```python
from build123d import *

# Parameters (mm, degrees)
SKETCH1_W               = 170
SKETCH1_H               = 80
SKETCH1_W_2             = 140
SKETCH1_H_2             = 50
BOSS_EXTRUDE1_DEPTH     = 20
CUT_EXTRUDE1_DEPTH      = 119.427192823
CUT_EXTRUDE1_DEPTH_BACK = 119.427192823
SKETCH2_R               = 6.3
CUT_EXTRUDE3_REACH      = 98.047
SKETCH5_R               = 2.75
FILLET1_R               = 2
FILLET2_R               = 5
SKETCH6_R               = 6
CUT_EXTRUDE4_DEPTH      = 119.427192823
SKETCH7_R               = 2.75
CUT_EXTRUDE5_DEPTH      = 97.046863561


with BuildPart() as part:
    # Sketch1 → Boss-Extrude1 (new body)
    with BuildSketch(Plane.XY):
        Rectangle(SKETCH1_W, SKETCH1_H)
        Rectangle(SKETCH1_W_2, SKETCH1_H_2, mode=Mode.SUBTRACT)
    extrude(amount=BOSS_EXTRUDE1_DEPTH)

    # Sketch2 → Cut-Extrude1 (cut, two sides: drawn at the far end of the back side and taken through both)
    with BuildSketch(Plane(origin=(0, 40, 0), x_dir=(1, 0, 0), z_dir=(0, 1, 0)).offset(-CUT_EXTRUDE1_DEPTH_BACK)):
        with Locations(Location((-60, -10, 0), (0, 0, 270))):
            Circle(SKETCH2_R)
        with Locations(Location((-10, -10, 0), (0, 0, 270))):
            Circle(SKETCH2_R)
    extrude(amount=CUT_EXTRUDE1_DEPTH + CUT_EXTRUDE1_DEPTH_BACK, mode=Mode.SUBTRACT)

    # Sketch5 → Cut-Extrude3 (cut, up to next)
    with BuildSketch(Plane(origin=(0, 0, 0), x_dir=(-1, 0, 0), z_dir=(0, 0, -1)), mode=Mode.PRIVATE) as cut_extrude3_sk1:
        with Locations((35, 32.5)):
            Circle(SKETCH5_R)
    cut_extrude3_tool1 = extrude(cut_extrude3_sk1.sketch, amount=-CUT_EXTRUDE3_REACH, mode=Mode.PRIVATE) & part.part
    # Sketch5 → Cut-Extrude3 (cut, up to next)
    with BuildSketch(Plane(origin=(0, 0, 0), x_dir=(-1, 0, 0), z_dir=(0, 0, -1)), mode=Mode.PRIVATE) as cut_extrude3_sk2:
        with Locations((35, -32.5)):
            Circle(SKETCH5_R)
    cut_extrude3_tool2 = extrude(cut_extrude3_sk2.sketch, amount=-CUT_EXTRUDE3_REACH, mode=Mode.PRIVATE) & part.part
    # Sketch5 → Cut-Extrude3 (cut, up to next)
    with BuildSketch(Plane(origin=(0, 0, 0), x_dir=(-1, 0, 0), z_dir=(0, 0, -1)), mode=Mode.PRIVATE) as cut_extrude3_sk3:
        with Locations((-5, 32.5)):
            Circle(SKETCH5_R)
    cut_extrude3_tool3 = extrude(cut_extrude3_sk3.sketch, amount=-CUT_EXTRUDE3_REACH, mode=Mode.PRIVATE) & part.part
    # Sketch5 → Cut-Extrude3 (cut, up to next)
    with BuildSketch(Plane(origin=(0, 0, 0), x_dir=(-1, 0, 0), z_dir=(0, 0, -1)), mode=Mode.PRIVATE) as cut_extrude3_sk4:
        with Locations((-5, -32.5)):
            Circle(SKETCH5_R)
    cut_extrude3_tool4 = extrude(cut_extrude3_sk4.sketch, amount=-CUT_EXTRUDE3_REACH, mode=Mode.PRIVATE) & part.part
    add(cut_extrude3_tool1.solids().sort_by_distance((-35, 32.5, 0))[0], mode=Mode.SUBTRACT)
    add(cut_extrude3_tool2.solids().sort_by_distance((-35, -32.5, 0))[0], mode=Mode.SUBTRACT)
    add(cut_extrude3_tool3.solids().sort_by_distance((5, 32.5, 0))[0], mode=Mode.SUBTRACT)
    add(cut_extrude3_tool4.solids().sort_by_distance((5, -32.5, 0))[0], mode=Mode.SUBTRACT)

    # Fillet1
    fillet1_edges = [part.edges().sort_by_distance(p)[0] for p in [
        (70, -25, 10),
        (70, 25, 10),
        (-70, 25, 10),
        (-70, -25, 10),
    ]]
    fillet(fillet1_edges, radius=FILLET1_R)

    # Fillet2
    fillet2_edges = [part.edges().sort_by_distance(p)[0] for p in [
        (85, -40, 10),
        (-85, -40, 10),
        (-85, 40, 10),
        (85, 40, 10),
    ]]
    fillet(fillet2_edges, radius=FILLET2_R)

    # Sketch6 → Cut-Extrude4 (cut, through all)
    with BuildSketch(Plane(origin=(0, 40, 0), x_dir=(1, 0, 0), z_dir=(0, 1, 0))):
        with Locations(Location((60, -10, 0), (0, 0, 270))):
            Circle(SKETCH6_R)
    extrude(amount=-CUT_EXTRUDE4_DEPTH, mode=Mode.SUBTRACT)

    # Sketch7 → Cut-Extrude5 (cut, through all)
    with BuildSketch(Plane(origin=(0, 0, 0), x_dir=(-1, 0, 0), z_dir=(0, 0, -1))):
        with Locations((-45, 32.5)):
            Circle(SKETCH7_R)
        with Locations((-45, -32.5)):
            Circle(SKETCH7_R)
    extrude(amount=-CUT_EXTRUDE5_DEPTH, mode=Mode.SUBTRACT)


solid = part.part
```
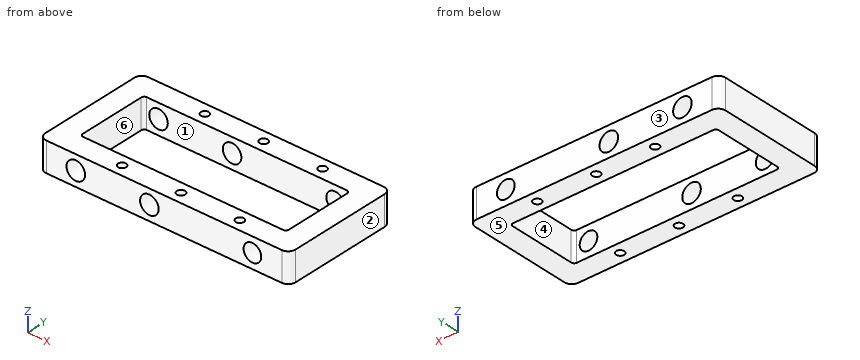
Check sheet for the modelled part. Datum: model origin and axes. Units: mm. Face numbers are marked on the shaded views. A direction names the side the tool comes from. Round coordinates to 2 decimals unless told otherwise and drop trailing zeros. Order: outer loops, then holes, each group sorted by start corner. A loop starts at its lowest first (then second) coordinate and runs counter-clockwise, first axis right, second up. Notation, with made-up numbers: (52, 57.5) -> (78, 57.5) arc R25 ccw to (78, 77.5) -> close; hole circle Ø3 at (-12, 74). An arc over 180 degrees is marked (long way). One line per item, written item: value. Start each with the question number.
Q1. Cross-section at A-A (y = -21). Record the boundary of the cut face in (x, z), and give its area (3 significant figures).
Q2. Thickness scan on line 1 (X direction, y = -29, z = 10.25); line 2 (Y direction, x = 45, z = 12.25); line 3 (X direction, y = 12, z = 6). Record the ranges inside material, lowest first.
Q3. Cross-section at B-B (x = 34). Record the boundary of the cut face in (y, z).
Q4. Set-up check for the marked faces 1 and 2: record each of +Z, -Z, +X, -X, +Y, -Y from which the full face is reachable in a straight line by a thin tool's end or side.
Q5. Cross-section at C-C (y = 32.5). Record the boundary of the cut face in (x, z), and give its area (3 significant figures).
Q6. Cross-section at D-D (x = 60). Record the boundary of the cut face in (y, z).
Q7. Gauge pin test, flat ends, axial feed: pin 1 Ø10 at (x, z) = (-10, 10) entering from -Y; pin 2 Ø8 at (x, y) = (40, -30.5) entering from -Z. Record the tip position at first contact, or that the pin passes through.
Q8. Mould release check, pull along Y, two halves, no side actions. Record for the marked faces 3, 4, 5 and 6: pulls with the +Y half, pulls with the -Y half, needs draft (parallel to the pull), parting line crosses it, or undercut.
Completed:
1. outline: (-85, 0) -> (-70, 0) -> (-70, 20) -> (-85, 20) -> close; (70, 0) -> (85, 0) -> (85, 20) -> (70, 20) -> close
1. area: 600 mm²
2. line 1: x = -85 to -66.3, -53.7 to -16.3, -3.7 to 54.01, 65.99 to 85
2. line 2: y = -40 to -35.25, -29.75 to -25, 25 to 29.75, 35.25 to 40
2. line 3: x = -85 to -70, 70 to 85
3. outline: (-40, 0) -> (-25, 0) -> (-25, 20) -> (-40, 20) -> close; (25, 0) -> (40, 0) -> (40, 20) -> (25, 20) -> close
4. face 1: +Z, -Z
4. face 2: +Z, -Z, +X, +Y, -Y
5. outline: (-85, 0) -> (-37.75, 0) -> (-37.75, 20) -> (-85, 20) -> close; (-32.25, 0) -> (2.25, 0) -> (2.25, 20) -> (-32.25, 20) -> close; (7.75, 0) -> (42.25, 0) -> (42.25, 20) -> (7.75, 20) -> close; (47.75, 0) -> (85, 0) -> (85, 20) -> (47.75, 20) -> close; hole circle Ø12.6 at (-60, 10); hole circle Ø12.6 at (-10, 10); hole circle Ø12 at (60, 10)
5. area: 2,710 mm²
6. outline: (-40, 0) -> (-25, 0) -> (-25, 4) -> (-40, 4) -> close; (-40, 16) -> (-25, 16) -> (-25, 20) -> (-40, 20) -> close; (25, 0) -> (40, 0) -> (40, 4) -> (25, 4) -> close; (25, 16) -> (40, 16) -> (40, 20) -> (25, 20) -> close
7. pin 1: passes through
7. pin 2: stops at z = 0
8. face 3: pulls with the +Y half
8. face 4: undercut
8. face 5: needs draft
8. face 6: undercut
